```python
from build123d import *

# Parameters (mm, degrees)
F1_DEPTH = 5
F1_TAPER = -15
F2_SIZE  = 2
F3_W     = 3.075
F3_H     = 5
F4_DEPTH = 5


with BuildPart() as f1:
    # F0 (on Top) → F1 (new body)
    with BuildSketch(Plane.XY):
        Polygon((-20, 8.2842712475), (-20, -8.2842712475), (-8.2842712475, -20), (8.2842712475, -20), (20, -8.2842712475), (20, 8.2842712475), (8.2842712475, 20), (-8.2842712475, 20), align=None)
    extrude(amount=F1_DEPTH, taper=F1_TAPER)

    # F2
    f2_edges = [f1.edges().sort_by_distance(p)[0] for p in [
        (-15.089479, -15.089479, 5),
        (0, -21.339746, 5),
        (15.089479, -15.089479, 5),
        (-21.339746, 0, 5),
        (-15.089479, 15.089479, 5),
        (21.339746, 0, 5),
        (15.089479, 15.089479, 5),
        (0, 21.339746, 5),
    ]]
    chamfer(f2_edges, length=F2_SIZE)

    # F3 (on face) → F4 (cut)
    with BuildSketch(Plane.XY.offset(5)):
        with Locations((1.5375, 0)):
            Rectangle(F3_W, F3_H)
    extrude(amount=-F4_DEPTH, mode=Mode.SUBTRACT)


solid = f1.part
```
Check sheet for the modelled part. Datum: model origin and axes. Units: mm. A direction names the side the tool comes from. Round coordinates to 2 decimals unless told otherwise and drop trailing zeros. Write item = value, one per line. Start each with the question number.
1. Gauge pin test, flat end, axial feed: pin 1 (3 mm diameter, centred on x = 3.5, z = 1, fed in from -Y). Record the tip position at first contact, or that the pin passes through.
2. Release check for a two-part mould opening along X. For faces 1 (the flat face through (2, 2.5, 3)), 2 (the flat face through (-0.4, -0.2, 5)) record: pulls with the +X half, pulls with the -X half, needs draft (parallel to the pull), parting line crosses it, or undercut.
3. Scan lines: line 1 (X direction, y = 0.5, z = 2.4) (3 decimals); line 2 (Y direction, x = 8.5, z = 3.05); line 3 (Y direction, x = -0.5, z = 0.2). Record each from-to range of solid material in increasing order. Write a range as [from, to].
4. Tool access check on faces 3 (the flat face through (-0.2, 0.4, 0)), 4 (the flat face through (0, 0, 3)). Record the directions out of +Z, -Z, +X, -X, +Y, -Y that give a thin tool (end or side, any length) a straight path to the whole face; none if there is none.
Results found:
q1.pin_1 = -20.67
q2.face_1 = undercut
q2.face_2 = needs draft
q3.line_1 = [-20.643, 0], [3.075, 20.643]
q3.line_2 = [-20.82, 20.82]
q3.line_3 = [-20.05, 20.05]
q4.face_3 = -Z, +X, -X, +Y, -Y
q4.face_4 = +Z, -Z
